```python
from build123d import *

# Parameters (mm, degrees)
ESQUISSE1_W             = 66
ESQUISSE1_H             = 127
BOSS_EXTRU_1_DEPTH      = 6
CONG_1_R                = 10
ESQUISSE2_R             = 1.5
ESQUISSE2_W             = 6
ESQUISSE2_H             = 67
ENL_V_MAT_EXTRU_1_DEPTH = 72.81399585
ESQUISSE5_R             = 2.995
ENL_V_MAT_EXTRU_4_DEPTH = 3


with BuildPart() as part:
    # Esquisse1 → Boss.-Extru.1 (new body)
    with BuildSketch(Plane.XY):
        Rectangle(ESQUISSE1_W, ESQUISSE1_H)
    extrude(amount=BOSS_EXTRU_1_DEPTH)

    # Congé1
    cong_1_edges = [part.edges().sort_by_distance(p)[0] for p in [
        (-33, -63.5, 3),
        (-33, 63.5, 3),
    ]]
    fillet(cong_1_edges, radius=CONG_1_R)

    # Esquisse2 → Enlèv. mat.-Extru.1 (cut, through all)
    with BuildSketch(Plane(origin=(0, 0, 0), x_dir=(-1, 0, 0), z_dir=(0, 0, -1))):
        with Locations((-30, -48.5)):
            Circle(ESQUISSE2_R)
        with Locations(Location((-30, 48.5, 0), (0, 0, 180))):
            Circle(ESQUISSE2_R)
        with Locations((-30, 0)):
            Rectangle(ESQUISSE2_W, ESQUISSE2_H)
    extrude(amount=-ENL_V_MAT_EXTRU_1_DEPTH, mode=Mode.SUBTRACT)

    # Esquisse5 → Enlèv. mat.-Extru.4 (cut)
    with BuildSketch(Plane.XY.offset(6)):
        with Locations((30, 48.5)):
            Circle(ESQUISSE5_R)
        with Locations((30, -48.5)):
            Circle(ESQUISSE5_R)
    extrude(amount=-ENL_V_MAT_EXTRU_4_DEPTH, mode=Mode.SUBTRACT)


solid = part.part
```
Part model, mm, in its own coordinate system. A direction names the side the tool comes from. Give positions to 0.01 mm unless a question says otherwise; leave off trailing zeros. Order: outer loops, then holes, each group sorted by start corner. A loop starts at its lowest first (then second) coordinate and runs counter-clockwise, first axis right, second up. Notation, with made-up numbers: M -0.75,-7 L 16.25,-7 A15 cw 16.25,19 Z; hole C 11.25,78.5 d1. An arc over 180 degrees is marked long. Use a Markdown table: item, result. Add a question column.
(1) Mould opens along Y. For faces 4 (the face through (31, 50, 3)), 5 (the face through (0, 1, 6)), 6 (the face through (5, -63.5, 3)), 7 (the face through (27, 0, 3)) say: +Y half, -Y half, draft (parallel to the pull), parting line (faces both ways), or undercut.
(2) Saw through at B-B, the plane x = 30. Give the cut face in (y, z) (3 decimals), and give its area (3 significant figures).
(3) Drop flat-ended pins along their axis: P1, Ø1.8, axis at y = -2.5, z = 3, coming from the +X side; P2, Ø3, axis at x = 29, y = 49, coming from the +Z side. Give the stop position or say it passes through.
(4) Probe line 1 along Y through (x, z) = (30, 2.25); line 2 along X through (y, z) = (10.5, 2.5); line 3 along Y through (x, z) = (-26.5, 5.6). List the from-to ranges inside material, lowest first. Write a range as [from, to].
(5) Saw through at A-A, the plane y = -48.5. Give the cut face in (x, z) (3 decimals).
(6) Saw through at D-D, the plane y = -19.5. Give the cut face in (x, z), and give its area (3 significant figures).
(7) 3-axis set-ups, long thin cutter, end or side, ignore diameter. For faces 1 (the face through (30, 50, 1)), 2 (the face through (29.61, 51.47, 4.52)), 3 (the face through (30, -33.5, 3)): which of +Z, -Z, +X, -X, +Y, -Y reach the whole face in a straight line?
(8) Saw through at C-C, the plane z = 4.1. Give the cut face in (x, y) (3 decimals), and give its area (3 significant figures).
Answer key:
| question | item | result |
|---|---|---|
| 1 | face 4 | undercut |
| 1 | face 5 | draft |
| 1 | face 6 | -Y half |
| 1 | face 7 | undercut |
| 2 | outline | M -63.5,0 L -50,0 L -50,3 L -51.495,3 L -51.495,6 L -63.5,6 Z; M -47,0 L -33.5,0 L -33.5,6 L -45.505,6 L -45.505,3 L -47,3 Z; M 33.5,0 L 47,0 L 47,3 L 45.505,3 L 45.505,6 L 33.5,6 Z; M 50,0 L 63.5,0 L 63.5,6 L 51.495,6 L 51.495,3 L 50,3 Z |
| 2 | area | 306 mm^2 |
| 3 | P1 | x = 27 |
| 3 | P2 | z = 3 |
| 4 | line 1 | [-63.5, -50], [-47, -33.5], [33.5, 47], [50, 63.5] |
| 4 | line 2 | [-33, 27] |
| 4 | line 3 | [-62.87, 62.87] |
| 5 | outline | M -33,0 L 28.5,0 L 28.5,3 L 27.005,3 L 27.005,6 L -33,6 Z; M 31.5,0 L 33,0 L 33,6 L 32.995,6 L 32.995,3 L 31.5,3 Z |
| 6 | outline | M -33,0 L 27,0 L 27,6 L -33,6 Z |
| 6 | area | 360 mm^2 |
| 7 | face 1 | +Z, -Z |
| 7 | face 2 | +Z |
| 7 | face 3 | +Z, -Z, +X |
| 8 | outline | M -33,-53.5 A10 ccw -23,-63.5 L 33,-63.5 L 33,-33.5 L 27,-33.5 L 27,33.5 L 33,33.5 L 33,63.5 L -23,63.5 A10 ccw -33,53.5 Z; hole C 30,-48.5 d5.99; hole C 30,48.5 d5.99 |
| 8 | area | 7,880 mm^2 |
